Autodesk Inventor part; units mm, degrees
ref_plane "b1_XY" through (-12.7, 0, -12.7) normal (1, 0, 0) x (0, 0, -1)
ref_plane "b1_YZ" through (-12.7, 0, -12.7) normal (0, 0, -1) x (0, 1, 0)
ref_plane "b1_ZX" through (-12.7, 0, -12.7) normal (0, 1, 0) x (1, 0, 0)
sketch "Sketch_1" plane through (0, 0, 0) normal (0, 0, 1) x (1, 0, 0)
  arc A0 (-12.6998, -10.5664) -> (-10.5664, -12.6998) centre (-10.5918, -10.5918) ccw
  arc A1 (-9.5504, -12.7) -> (-10.5664, -12.6998) centre (-10.0584, -12.7) ccw
  line L0 (-9.5504, -12.7) -> (-6.3331, -12.7)
  arc A2 (-5.3171, -12.7) -> (-6.3331, -12.7) centre (-5.8251, -12.7) ccw
  line L1 (-5.3171, -12.7) -> (-4.3434, -12.7)
  arc A3 (-4.3434, -12.7) -> (-4.3434, -10.4902) centre (-4.3434, -11.5951) ccw
  line L2 (-4.3434, -10.4902) -> (-6.4748, -10.4902)
  arc A4 (-7.1932, -8.7558) -> (-6.4748, -10.4902) centre (-6.4748, -9.4742) ccw
  line L3 (-7.1932, -8.7558) -> (-3.8632, -5.4257)
  arc A5 (-1.6181, -4.4958) -> (-3.8632, -5.4257) centre (-1.6181, -7.6708) ccw
  line L4 (-1.6181, -4.4958) -> (1.6181, -4.4958)
  arc A6 (3.8632, -5.4257) -> (1.6181, -4.4958) centre (1.6181, -7.6708) ccw
  line L5 (3.8632, -5.4257) -> (7.1932, -8.7558)
  arc A7 (6.4748, -10.4902) -> (7.1932, -8.7558) centre (6.4748, -9.4742) ccw
  line L6 (6.4748, -10.4902) -> (4.3434, -10.4902)
  arc A8 (4.3434, -10.4902) -> (4.3434, -12.7) centre (4.3434, -11.5951) ccw
  line L7 (4.3434, -12.7) -> (5.3171, -12.7)
  arc A9 (6.3331, -12.7) -> (5.3171, -12.7) centre (5.8251, -12.7) ccw
  line L8 (6.3331, -12.7) -> (9.5504, -12.7)
  arc A10 (10.5664, -12.6998) -> (9.5504, -12.7) centre (10.0584, -12.7) ccw
  arc A11 (10.5664, -12.6998) -> (12.6998, -10.5664) centre (10.5918, -10.5918) ccw
  arc A12 (12.7, -9.5504) -> (12.6998, -10.5664) centre (12.7, -10.0584) ccw
  line L9 (12.7, -9.5504) -> (12.7, -6.3331)
  arc A13 (12.7, -5.3171) -> (12.7, -6.3331) centre (12.7, -5.8251) ccw
  line L10 (12.7, -5.3171) -> (12.7, -4.3434)
  arc A14 (12.7, -4.3434) -> (10.4902, -4.3434) centre (11.5951, -4.3434) ccw
  line L11 (10.4902, -4.3434) -> (10.4902, -6.4748)
  arc A15 (8.7558, -7.1932) -> (10.4902, -6.4748) centre (9.4742, -6.4748) ccw
  line L12 (8.7558, -7.1932) -> (5.4257, -3.8632)
  arc A16 (4.4958, -1.6181) -> (5.4257, -3.8632) centre (7.6708, -1.6181) ccw
  line L13 (4.4958, -1.6181) -> (4.4958, 1.6181)
  arc A17 (5.4257, 3.8632) -> (4.4958, 1.6181) centre (7.6708, 1.6181) ccw
  line L14 (5.4257, 3.8632) -> (8.7558, 7.1932)
  arc A18 (10.4902, 6.4748) -> (8.7558, 7.1932) centre (9.4742, 6.4748) ccw
  line L15 (10.4902, 6.4748) -> (10.4902, 4.3434)
  arc A19 (10.4902, 4.3434) -> (12.7, 4.3434) centre (11.5951, 4.3434) ccw
  line L16 (12.7, 4.3434) -> (12.7, 5.3171)
  arc A20 (12.7, 6.3331) -> (12.7, 5.3171) centre (12.7, 5.8251) ccw
  line L17 (12.7, 6.3331) -> (12.7, 9.5504)
  arc A21 (12.6998, 10.5664) -> (12.7, 9.5504) centre (12.7, 10.0584) ccw
  arc A22 (12.6998, 10.5664) -> (10.5664, 12.6998) centre (10.5918, 10.5918) ccw
  arc A23 (9.5504, 12.7) -> (10.5664, 12.6998) centre (10.0584, 12.7) ccw
  line L18 (9.5504, 12.7) -> (6.3331, 12.7)
  arc A24 (5.3171, 12.7) -> (6.3331, 12.7) centre (5.8251, 12.7) ccw
  line L19 (5.3171, 12.7) -> (4.3434, 12.7)
  arc A25 (4.3434, 12.7) -> (4.3434, 10.4902) centre (4.3434, 11.5951) ccw
  line L20 (4.3434, 10.4902) -> (6.4748, 10.4902)
  arc A26 (7.1932, 8.7558) -> (6.4748, 10.4902) centre (6.4748, 9.4742) ccw
  line L21 (7.1932, 8.7558) -> (3.8632, 5.4257)
  arc A27 (1.6181, 4.4958) -> (3.8632, 5.4257) centre (1.6181, 7.6708) ccw
  line L22 (1.6181, 4.4958) -> (-1.6181, 4.4958)
  arc A28 (-3.8632, 5.4257) -> (-1.6181, 4.4958) centre (-1.6181, 7.6708) ccw
  line L23 (-3.8632, 5.4257) -> (-7.1932, 8.7558)
  arc A29 (-6.4748, 10.4902) -> (-7.1932, 8.7558) centre (-6.4748, 9.4742) ccw
  line L24 (-6.4748, 10.4902) -> (-4.3434, 10.4902)
  arc A30 (-4.3434, 10.4902) -> (-4.3434, 12.7) centre (-4.3434, 11.5951) ccw
  line L25 (-4.3434, 12.7) -> (-5.3171, 12.7)
  arc A31 (-6.3331, 12.7) -> (-5.3171, 12.7) centre (-5.8251, 12.7) ccw
  line L26 (-6.3331, 12.7) -> (-9.5504, 12.7)
  arc A32 (-10.5664, 12.6998) -> (-9.5504, 12.7) centre (-10.0584, 12.7) ccw
  arc A33 (-10.5664, 12.6998) -> (-12.6998, 10.5664) centre (-10.5918, 10.5918) ccw
  arc A34 (-12.7, 9.5504) -> (-12.6998, 10.5664) centre (-12.7, 10.0584) ccw
  line L27 (-12.7, 9.5504) -> (-12.7, 6.3331)
  arc A35 (-12.7, 5.3171) -> (-12.7, 6.3331) centre (-12.7, 5.8251) ccw
  line L28 (-12.7, 5.3171) -> (-12.7, 4.3434)
  arc A36 (-12.7, 4.3434) -> (-10.4902, 4.3434) centre (-11.5951, 4.3434) ccw
  line L29 (-10.4902, 4.3434) -> (-10.4902, 6.4748)
  arc A37 (-8.7558, 7.1932) -> (-10.4902, 6.4748) centre (-9.4742, 6.4748) ccw
  line L30 (-8.7558, 7.1932) -> (-5.4257, 3.8632)
  arc A38 (-4.4958, 1.6181) -> (-5.4257, 3.8632) centre (-7.6708, 1.6181) ccw
  line L31 (-4.4958, 1.6181) -> (-4.4958, -1.6181)
  arc A39 (-5.4257, -3.8632) -> (-4.4958, -1.6181) centre (-7.6708, -1.6181) ccw
  line L32 (-5.4257, -3.8632) -> (-8.7558, -7.1932)
  arc A40 (-10.4902, -6.4748) -> (-8.7558, -7.1932) centre (-9.4742, -6.4748) ccw
  line L33 (-10.4902, -6.4748) -> (-10.4902, -4.3434)
  arc A41 (-10.4902, -4.3434) -> (-12.7, -4.3434) centre (-11.5951, -4.3434) ccw
  line L34 (-12.7, -4.3434) -> (-12.7, -5.3171)
  arc A42 (-12.7, -6.3331) -> (-12.7, -5.3171) centre (-12.7, -5.8251) ccw
  line L35 (-12.7, -6.3331) -> (-12.7, -9.5504)
  arc A43 (-12.6998, -10.5664) -> (-12.7, -9.5504) centre (-12.7, -10.0584) ccw
  circle A44 centre (0, 0) radius 2.6035
extrude "Extrusion1" add sketch "Sketch_1" against normal blind 160
ref_plane "b1_XY" through (-12.7, 0, -12.7) normal (1, 0, 0) x (0, 0, -1)
ref_plane "b1_YZ" through (-12.7, 0, -12.7) normal (0, 0, -1) x (0, 1, 0)
ref_plane "b1_ZX" through (-12.7, 0, -12.7) normal (0, 1, 0) x (1, 0, 0)
ref_plane "b2_XY" through (12.7, 0, -12.7) normal (1, 0, 0) x (0, 0, -1)
ref_plane "b2_YZ" through (12.7, 0, -12.7) normal (0, 0, -1) x (0, 1, 0)
ref_plane "b2_ZX" through (12.7, 0, -12.7) normal (0, 1, 0) x (1, 0, 0)
ref_plane "profile1010_XY" through (0, 0, -12.7) normal (0, 0, 1) x (1, 0, 0)
ref_plane "profile1010_YZ" through (0, 0, -12.7) normal (1, 0, 0) x (0, 1, 0)
ref_plane "profile1010_ZX" through (0, 0, -12.7) normal (0, 1, 0) x (0, 0, 1)
properties part number "1010_160mm"
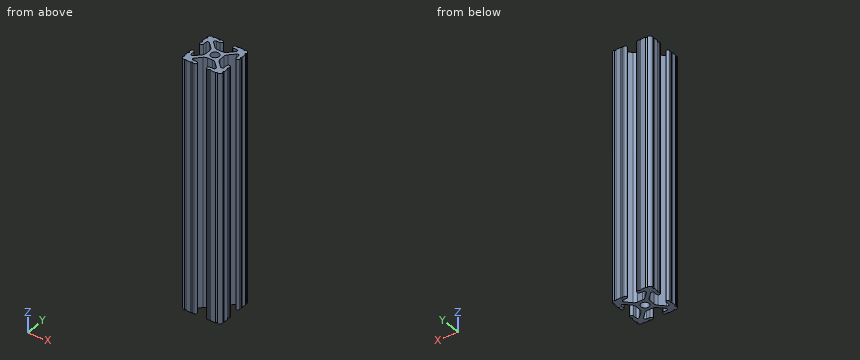
Build history of the part. All positions in model axes, mm. Coordinates: 2 decimals unless noted, no trailing zeros. Write each loop counter-clockwise with the first axis right and the second up, starting at its lowest first coordinate (ties: lowest second). Pieces come first, ordered by that corner, then holes.
(1) Cut at A-A on x = 0. List the corners of the cut face in (y, z), and give its area (3 significant figures).
(2) Drill centre lines: line 1 (Y direction, x = 0, z = -79); line 2 (X direction, y = -3.5, z = -95); line 3 (X direction, y = -4, z = -117). Where is each one in solid material? Low to high.
(3) Pin check, flat tips, straight feed: pin 1 Ø1.6 at (y, z) = (0, -77) entering from +X; pin 2 Ø2.5 at (x, z) = (-0.5, -109) entering from +Y; pin 3 Ø1 at (y, z) = (0, -106.5) entering from -X. Stop position of each tip, or through.
Working result:
1. outline: (-4.5, -160) - (-2.6, -160) - (-2.6, 0) - (-4.5, 0) - close; (2.6, -160) - (4.5, -160) - (4.5, 0) - (2.6, 0) - close
1. area: 606 mm2
2. line 1: y = -4.5 to -2.6, 2.6 to 4.5
2. line 2: x = -12.31 to -10.88, -5.11 to 5.11, 10.88 to 12.31
2. line 3: x = -12.65 to -10.54, -5.56 to 5.56, 10.54 to 12.65
3. pin 1: stops at x = 4.5
3. pin 2: stops at y = 4.5
3. pin 3: stops at x = -4.5
